from build123d import *

# Parameters (mm, degrees)
EXTRUDE_1_DEPTH          = 5
SKETCH_2_R               = 1.45
CUT_EXTRUDE_1_DEPTH      = 5
SKETCH_3_R               = 1.475
CUT_EXTRUDE_2_DEPTH      = 46
PATTERN_CIRCULAR_1_COUNT = 2
PATTERN_CIRCULAR_1_ANGLE = 35
MIRROR_1_COPY_1_SKETCH_R = 1.475
MIRROR_1_COPY_1_DEPTH    = 46


with BuildPart() as part:
    # Sketch 1 → Extrude 1 (new body)
    with BuildSketch(Plane(origin=(0, 0, 0), x_dir=(1, 0, 0), z_dir=(0, 1, 0))):
        with BuildLine():
            Line((27.395437576, 29.146011734), (27.395437576, 35.7))
            ThreePointArc((27.395437576, 35.7), (45, 0), (27.395437576, -35.7))
            Line((27.395437576, -35.7), (27.395437576, -29.146011734))
            ThreePointArc((27.395437576, -29.146011734), (40, 0), (27.395437576, 29.146011734))
        make_face()
    extrude(amount=EXTRUDE_1_DEPTH)

    # Sketch 2 → Cut-Extrude 1 (cut)
    with BuildSketch(Plane(origin=(0, 5, 0), x_dir=(1, 0, 0), z_dir=(0, 1, 0))):
        with Locations(Location((42.5, 0, 0), (0, 0, 270))):
            Circle(SKETCH_2_R)
        with Locations(Location((32.556888833, 27.318473412, 0), (0, 0, 270))):
            Circle(SKETCH_2_R)
        with Locations(Location((32.556888833, -27.318473412, 0), (0, 0, 90))):
            Circle(SKETCH_2_R)
    extrude(amount=-CUT_EXTRUDE_1_DEPTH, mode=Mode.SUBTRACT)

    # Sketch 3 → Cut-Extrude 2 (cut)
    with BuildSketch(Plane(origin=(0, 0, 0), x_dir=(0, 1, 0), z_dir=(0.7193398003386524, 0, 0.6946583704589961))):
        with Locations(Location((2.5, 0, 0), (0, 0, 90))):
            Circle(SKETCH_3_R)
    cut_extrude_2 = extrude(amount=CUT_EXTRUDE_2_DEPTH, mode=Mode.SUBTRACT)

    # Pattern Circular 1: Cut-Extrude 2 ×2 about axis
    pattern_circular_1_axis = Axis((0, -0.25, 0), (0, 1, 0))
    for i in range(1, PATTERN_CIRCULAR_1_COUNT):
        add(cut_extrude_2.rotate(pattern_circular_1_axis, i * PATTERN_CIRCULAR_1_ANGLE / (PATTERN_CIRCULAR_1_COUNT - 1)), mode=Mode.SUBTRACT)

    # Mirror 1: Cut-Extrude 2 across plane
    add(cut_extrude_2.mirror(Plane.XY), mode=Mode.SUBTRACT)

    # Mirror 1 copy 1 sketch → Mirror 1 copy 1 (cut)
    with BuildSketch(Plane(origin=(0, 0, 0), x_dir=(0, 1, 0), z_dir=(0.9876883405951382, 0, -0.15643446504022812))):
        with Locations((2.5, 0)):
            Circle(MIRROR_1_COPY_1_SKETCH_R)
    extrude(amount=MIRROR_1_COPY_1_DEPTH, mode=Mode.SUBTRACT)


solid = part.part
The listing builds one solid part. Answer for the finished solid, in the listing's coordinates (mm). Give positions to 0.01 mm unless a question says otherwise; leave off trailing zeros. Order: outer loops, then holes, each group sorted by start corner. A loop starts at its lowest first (then second) coordinate and runs counter-clockwise, first axis right, second up. Notation, with made-up numbers: (51, 6.5) - (55, 6.5) arc R15 ccw to (55, 31.5) - close; hole circle Ø10 at (88, 0). An arc over 180 degrees is marked (long way). One line per item, written item: value. Start each with the question number.
1) A cutting plane is placed at B-B on x = 42.5. State how many separate pieces and enclosed holes the cut face has, then the cut area to 3 significant figures.
2) Find the intervals of material crossed by L1, parallel to Z at x = 33, y = 0.5; L2, parallel to Z at x = 40.75, y = 1.5; L3, parallel to Z at x = 28.5, y = 3.1, in increasing order.
3) The mould has two halves that part along X. Classify faces 1 (the face through (30.67, 1.038, -29.351)), 2 (the face through (41, 5, 2)), 3 (the face through (31.12, 2.54, 27.51)), 4 (the face through (27.395, 2, -32)): released by +X, released by -X, zero draft, split by the parting line, or undercut.
4) Given pin 1 Ø2.5 at (x, z) = (42.5, 0) entering from +Y; pin 2 Ø4 at (x, z) = (32.56, 27.32) entering from -Y; pin 3 Ø2 at (x, y) = (39, 2) entering from -Z; pin 4 Ø3 at (x, y) = (41, 2) entering from -Z, each flat-ended and moving along its own axis, determine where each tip first touches the part or whether it passes through.
5) A cutting plane is placed at C-C on z = 17.5. Give the vertices of the cut face in (x, y), then the cut area to 3 significant figures.
6) A cutting plane is placed at A-A on z = 0. Give the vertices of the cut face in (x, y), then the cut area to 3 significant figures.
Answer sheet:
1. separate pieces: 2
1. enclosed holes: 2
1. area: 120 mm2
2. L1: z = -30.59 to -28.7, -25.94 to -22.61, 22.61 to 25.94, 28.7 to 30.59
2. L2: z = -19.09 to -7.55, -5.36 to 5.36, 7.55 to 19.09
2. L3: z = -34.82 to -29.4, 29.4 to 34.82
3. face 1: undercut
3. face 2: zero draft
3. face 3: undercut
3. face 4: released by -X
4. pin 1: passes through
4. pin 2: stops at y = 0
4. pin 3: stops at z = -24.1
4. pin 4: stops at z = -21.56
5. outline: (35.97, 0) - (41.46, 0) - (41.46, 5) - (35.97, 5) - close
5. area: 27.4 mm2
6. outline: (40, 0) - (41.05, 0) - (41.05, 5) - (40, 5) - close; (43.95, 0) - (45, 0) - (45, 5) - (43.95, 5) - close
6. area: 10.5 mm2
